Model file for the job. Use its own axes, mm. Give positions to 0.01 mm unless a question says otherwise; leave off trailing zeros. Loops run counter-clockwise (first coordinate to the right, second up) from the corner with the lowest first, then second, coordinate; pieces in that order, holes last. Notation, with made-up numbers: (57, 5.5) - (110, 5.5) arc R23 ccw to (110, 39.5) - close; hole circle Ø8 at (-23.75, 80.5). An arc over 180 degrees is marked (long way). Use a Markdown table: item, result.
from build123d import *

# Parameters (mm, degrees)
SKETCH1_R           = 1.5
SKETCH1_R_2         = 3
SKETCH1_R_3         = 2
SKETCH1_W           = 12.75
SKETCH1_H           = 8.25
BOSS_EXTRUDE1_DEPTH = 2
FILLET1_R           = 1.5


with BuildPart() as part:
    # Sketch1 → Boss-Extrude1 (new body)
    with BuildSketch(Plane(origin=(0, 0, 0), x_dir=(1, 0, 0), z_dir=(0, 1, 0))):
        Polygon((0, 20), (0, 104), (12, 104), (14, 93), (26, 93), (26, 107), (33.5, 114), (62.5, 114), (70, 107), (70, 93), (82, 93), (84, 104), (96, 104), (96, 20), (89, 9), (89, 0), (62, 0), (62, 8), (34, 8), (34, 0), (7, 0), (7, 9), align=None)
        with Locations(Location((12.5, 3, 0), (0, 0, 270))):
            Circle(SKETCH1_R, mode=Mode.SUBTRACT)
        with Locations(Location((28, 3, 0), (0, 0, 270))):
            Circle(SKETCH1_R, mode=Mode.SUBTRACT)
        with Locations(Location((68, 3, 0), (0, 0, 90))):
            Circle(SKETCH1_R, mode=Mode.SUBTRACT)
        with Locations(Location((83.5, 3, 0), (0, 0, 90))):
            Circle(SKETCH1_R, mode=Mode.SUBTRACT)
        with Locations(Location((14, 13, 0), (0, 0, 270))):
            Circle(SKETCH1_R_2, mode=Mode.SUBTRACT)
        with Locations(Location((27, 13, 0), (0, 0, 270))):
            Circle(SKETCH1_R_2, mode=Mode.SUBTRACT)
        with Locations(Location((69, 13, 0), (0, 0, 90))):
            Circle(SKETCH1_R_2, mode=Mode.SUBTRACT)
        with Locations(Location((82, 13, 0), (0, 0, 90))):
            Circle(SKETCH1_R_2, mode=Mode.SUBTRACT)
        with Locations(Location((22.75, 42.455027657, 0), (0, 0, 270))):
            Circle(SKETCH1_R, mode=Mode.SUBTRACT)
        with Locations(Location((22.75, 51.751081058, 0), (0, 0, 270))):
            Circle(SKETCH1_R, mode=Mode.SUBTRACT)
        with Locations(Location((73.25, 42.455027657, 0), (0, 0, 90))):
            Circle(SKETCH1_R, mode=Mode.SUBTRACT)
        with Locations(Location((73.25, 51.751081058, 0), (0, 0, 90))):
            Circle(SKETCH1_R, mode=Mode.SUBTRACT)
        with Locations(Location((18, 72.75, 0), (0, 0, 270))):
            Circle(SKETCH1_R, mode=Mode.SUBTRACT)
        with Locations(Location((28, 65.75, 0), (0, 0, 270))):
            Circle(SKETCH1_R, mode=Mode.SUBTRACT)
        with Locations(Location((68, 65.75, 0), (0, 0, 90))):
            Circle(SKETCH1_R, mode=Mode.SUBTRACT)
        with Locations(Location((78, 72.75, 0), (0, 0, 90))):
            Circle(SKETCH1_R, mode=Mode.SUBTRACT)
        with Locations(Location((36.5, 76.75, 0), (0, 0, 270))):
            Circle(SKETCH1_R_3, mode=Mode.SUBTRACT)
        with Locations(Location((59.5, 76.75, 0), (0, 0, 90))):
            Circle(SKETCH1_R_3, mode=Mode.SUBTRACT)
        with Locations(Location((35.5, 89, 0), (0, 0, 270))):
            Circle(SKETCH1_R, mode=Mode.SUBTRACT)
        with Locations(Location((35.5, 106.5, 0), (0, 0, 270))):
            Circle(SKETCH1_R, mode=Mode.SUBTRACT)
        with Locations(Location((60.5, 89, 0), (0, 0, 90))):
            Circle(SKETCH1_R, mode=Mode.SUBTRACT)
        with Locations(Location((60.5, 106.5, 0), (0, 0, 90))):
            Circle(SKETCH1_R, mode=Mode.SUBTRACT)
        with Locations(Location((44, 26, 0), (0, 0, 270))):
            Circle(SKETCH1_R, mode=Mode.SUBTRACT)
        with Locations(Location((52, 26, 0), (0, 0, 90))):
            Circle(SKETCH1_R, mode=Mode.SUBTRACT)
        with Locations(Location((52, 74, 0), (0, 0, 270))):
            Circle(SKETCH1_R, mode=Mode.SUBTRACT)
        with Locations(Location((44, 74, 0), (0, 0, 90))):
            Circle(SKETCH1_R, mode=Mode.SUBTRACT)
        with Locations(Location((48, 97.75, 0), (0, 0, 270))):
            Circle(SKETCH1_R_3, mode=Mode.SUBTRACT)
        with Locations((69.875, 25.875)):
            Rectangle(SKETCH1_W, SKETCH1_H, mode=Mode.SUBTRACT)
        with Locations((26.125, 25.875)):
            Rectangle(SKETCH1_W, SKETCH1_H, mode=Mode.SUBTRACT)
        with Locations((69.875, 81.875)):
            Rectangle(SKETCH1_W, SKETCH1_H, mode=Mode.SUBTRACT)
        with Locations((26.125, 81.875)):
            Rectangle(SKETCH1_W, SKETCH1_H, mode=Mode.SUBTRACT)
        with BuildLine():
            Line((3, 75), (7, 75))
            ThreePointArc((7, 75), (9, 73), (7, 71))
            Line((7, 71), (3, 71))
            ThreePointArc((3, 71), (1, 73), (3, 75))
        make_face(mode=Mode.SUBTRACT)
        with BuildLine():
            Line((93, 75), (89, 75))
            ThreePointArc((89, 75), (87, 73), (89, 71))
            Line((89, 71), (93, 71))
            ThreePointArc((93, 71), (95, 73), (93, 75))
        make_face(mode=Mode.SUBTRACT)
        with BuildLine():
            Line((93, 37), (89, 37))
            ThreePointArc((89, 37), (87, 35), (89, 33))
            Line((89, 33), (93, 33))
            ThreePointArc((93, 33), (95, 35), (93, 37))
        make_face(mode=Mode.SUBTRACT)
        with BuildLine():
            Line((3, 33), (7, 33))
            ThreePointArc((7, 33), (9, 35), (7, 37))
            Line((7, 37), (3, 37))
            ThreePointArc((3, 37), (1, 35), (3, 33))
        make_face(mode=Mode.SUBTRACT)
        with BuildLine():
            Line((15, 48.525154469), (23, 48.525154469))
            ThreePointArc((23, 48.525154469), (24.5, 47.025154469), (23, 45.525154469))
            Line((23, 45.525154469), (15, 45.525154469))
            ThreePointArc((15, 45.525154469), (13.5, 47.025154469), (15, 48.525154469))
        make_face(mode=Mode.SUBTRACT)
        with BuildLine():
            Line((81, 48.525154469), (73, 48.525154469))
            ThreePointArc((73, 48.525154469), (71.5, 47.025154469), (73, 45.525154469))
            Line((73, 45.525154469), (81, 45.525154469))
            ThreePointArc((81, 45.525154469), (82.5, 47.025154469), (81, 48.525154469))
        make_face(mode=Mode.SUBTRACT)
        with BuildLine():
            Line((16.5, 67.75), (16.5, 57.75))
            ThreePointArc((16.5, 57.75), (18, 56.25), (19.5, 57.75))
            Line((19.5, 57.75), (19.5, 67.75))
            ThreePointArc((19.5, 67.75), (18, 69.25), (16.5, 67.75))
        make_face(mode=Mode.SUBTRACT)
        with BuildLine():
            Line((76.5, 67.75), (76.5, 57.75))
            ThreePointArc((76.5, 57.75), (78, 56.25), (79.5, 57.75))
            Line((79.5, 57.75), (79.5, 67.75))
            ThreePointArc((79.5, 67.75), (78, 69.25), (76.5, 67.75))
        make_face(mode=Mode.SUBTRACT)
        with BuildLine():
            Line((46.5, 29), (38, 29))
            Line((38, 29), (38, 71))
            Line((38, 71), (46.5, 71))
            Line((46.5, 71), (46.5, 74))
            ThreePointArc((46.5, 74), (48, 75.5), (49.5, 74))
            Line((49.5, 74), (49.5, 71))
            Line((49.5, 71), (58, 71))
            Line((58, 71), (58, 29))
            Line((58, 29), (49.5, 29))
            Line((49.5, 29), (49.5, 26))
            ThreePointArc((49.5, 26), (48, 24.5), (46.5, 26))
            Line((46.5, 26), (46.5, 29))
        make_face(mode=Mode.SUBTRACT)
    extrude(amount=BOSS_EXTRUDE1_DEPTH)

    # Fillet1
    fillet1_edges = [part.edges().sort_by_distance(p)[0] for p in [
        (19.75, 1, -30),
        (19.75, 1, -21.75),
        (32.5, 1, -21.75),
        (32.5, 1, -30),
        (63.5, 1, -77.75),
        (76.25, 1, -77.75),
        (76.25, 1, -86),
        (63.5, 1, -86),
        (19.75, 1, -86),
        (19.75, 1, -77.75),
        (32.5, 1, -77.75),
        (32.5, 1, -86),
        (58, 1, -29),
        (58, 1, -71),
        (38, 1, -71),
        (38, 1, -29),
        (62, 1, -8),
        (34, 1, -8),
        (34, 1, 0),
        (7, 1, 0),
        (7, 1, -9),
        (0, 1, -20),
        (0, 1, -104),
        (12, 1, -104),
        (14, 1, -93),
        (26, 1, -93),
        (26, 1, -107),
        (33.5, 1, -114),
        (62.5, 1, -114),
        (70, 1, -107),
        (70, 1, -93),
        (82, 1, -93),
        (84, 1, -104),
        (96, 1, -104),
        (96, 1, -20),
        (89, 1, -9),
        (89, 1, 0),
        (62, 1, 0),
        (76.25, 1, -21.75),
        (76.25, 1, -30),
        (63.5, 1, -30),
        (63.5, 1, -21.75),
    ]]
    fillet(fillet1_edges, radius=FILLET1_R)


solid = part.part
(1) Pin check, flat tips, straight feed: P1, Ø1, axis at y = 0.5, z = -5, coming from the -X side; P2, Ø6, axis at x = 84, z = -13.5, coming from the +Y side. Stop position of each tip, or through.
Computed:
| item | result |
|---|---|
| P1 | x = 7 |
| P2 | y = 2 |
(2) Slice it at B-B, the plane z = -80.5. Write the cut outline in (x, y), plus the area to 3 significant figures.
Computed:
| item | result |
|---|---|
| outline | (0, 0) - (19.75, 0) - (19.75, 2) - (0, 2) - close; (32.5, 0) - (63.5, 0) - (63.5, 2) - (32.5, 2) - close; (76.25, 0) - (96, 0) - (96, 2) - (76.25, 2) - close |
| area | 141 mm² |
(3) Slice it at A-A, the plane x = 44. Write the cut outline in (y, z), plus the area to 3 significant figures.
Computed:
| item | result |
|---|---|
| outline | (0, -114) - (2, -114) - (2, -75.5) - (0, -75.5) - close; (0, -72.5) - (2, -72.5) - (2, -71) - (0, -71) - close; (0, -29) - (2, -29) - (2, -27.5) - (0, -27.5) - close; (0, -24.5) - (2, -24.5) - (2, -8) - (0, -8) - close |
| area | 116 mm² |
(4) Slice it at D-D, the plane z = -97.75. Write the cut outline in (x, y).
Computed:
| item | result |
|---|---|
| outline | (0, 0) - (13.14, 0) - (13.14, 2) - (0, 2) - close; (26, 0) - (46, 0) - (46, 2) - (26, 2) - close; (50, 0) - (70, 0) - (70, 2) - (50, 2) - close; (82.86, 0) - (96, 0) - (96, 2) - (82.86, 2) - close |
(5) Slice it at C-C, the plane z = -3. Write the cut outline in (x, y), plus the area to 3 significant figures.
Computed:
| item | result |
|---|---|
| outline | (7, 0) - (11, 0) - (11, 2) - (7, 2) - close; (14, 0) - (26.5, 0) - (26.5, 2) - (14, 2) - close; (29.5, 0) - (34, 0) - (34, 2) - (29.5, 2) - close; (62, 0) - (66.5, 0) - (66.5, 2) - (62, 2) - close; (69.5, 0) - (82, 0) - (82, 2) - (69.5, 2) - close; (85, 0) - (89, 0) - (89, 2) - (85, 2) - close |
| area | 84.0 mm² |
(6) Mould opens along X. For faces 1 (the flat face through (59, 2, -58)), 2 (the cylindrical face through (45.33, 0.99, -74.69)), 3 (the flat face through (29.73, 0.99, -110.48)), 4 (the flat face through (66.182, 0.986, -110.564)) say: pulls with the +X half, pulls with the -X half, needs draft (parallel to the pull), parting line crosses it, or undercut.
Computed:
| item | result |
|---|---|
| face 1 | needs draft |
| face 2 | undercut |
| face 3 | pulls with the -X half |
| face 4 | pulls with the +X half |
(7) Drill centre lines: probe 1 along Z at (x, y) = (73.5, 1.6); probe 2 along Z at (x, y) = (73.25, 1.25); probe 3 along X at (y, z) = (1.65, -26). Where is each one in solid material? Low to high. Write a range as [from, to].
Computed:
| item | result |
|---|---|
| probe 1 | [-93, -86], [-77.75, -53.23], [-50.27, -48.53], [-45.53, -43.93], [-40.98, -30], [-21.75, 0] |
| probe 2 | [-93, -86], [-77.75, -53.25], [-50.25, -48.53], [-45.53, -43.96], [-40.96, -30], [-21.75, 0] |
| probe 3 | [0, 19.75], [32.5, 42.5], [45.5, 46.5], [49.5, 50.5], [53.5, 63.5], [76.25, 96] |
